from build123d import *

# Parameters (mm, degrees)
SKETCH1_W           = 820
SKETCH1_H           = 210
BOSS_EXTRUDE1_DEPTH = 210
CUT_EXTRUDE5_DEPTH  = 336
BOSS_EXTRUDE2_DEPTH = 210
BOSS_EXTRUDE3_DEPTH = 5
BOSS_EXTRUDE4_DEPTH = 5
SHELL2_START        = 5
SHELL2_DEPTH        = 200


# Read off the part's stored shape, not the designer's step: Shell2
with BuildPart() as part:
    # Sketch1 → Boss-Extrude1 (new body)
    with BuildSketch(Plane.XY):
        Rectangle(SKETCH1_W, SKETCH1_H)
    extrude(amount=BOSS_EXTRUDE1_DEPTH)

    # Sketch2 → Cut-Extrude5 (cut)
    with BuildSketch(Plane.XY.offset(210)):
        Polygon((-409.131759112, -82.443263164), (-310, -99.922866941), (-310, 99.822096903), (-310.868240888, 100.075961235), (-338.793852416, 105), (-410, 105), (-410, -82.367301929), align=None)
        Polygon((-410, -105), (-310, -105), (-410, -87.367301929), align=None)
    extrude(amount=-CUT_EXTRUDE5_DEPTH, mode=Mode.SUBTRACT)

    # Sketch6 → Boss-Extrude2 (add, through all)
    with BuildSketch(Plane.XY.offset(210)):
        Polygon((-338.793852416, 105), (-310.434120444, 105), (-410.434120444, 122.632698071), (-410.434120444, 117.555565011), (-311.302361333, 100.075961235), (-310.434120444, 99.437059413), (-310.434120444, 99.949029069), (-310.868240888, 100.075961235), align=None)
    extrude(amount=-BOSS_EXTRUDE2_DEPTH)

    # Sketch8 → Boss-Extrude3 (add)
    with BuildSketch(Plane.XY.offset(210)):
        Polygon((-410, -87.367301929), (-310, -105), (410, -105), (410, 105), (-310.434120444, 105), (-410.434120444, 122.632698071), align=None)
    extrude(amount=-BOSS_EXTRUDE3_DEPTH)

    # Sketch9 → Boss-Extrude4 (add)
    with BuildSketch(Plane(origin=(0, 0, 0), x_dir=(-1, 0, 0), z_dir=(0, 0, -1))):
        Polygon((310.434120444, 105), (310, -105), (410, -87.367301929), (410.434120444, 122.632698071), align=None)
    extrude(amount=-BOSS_EXTRUDE4_DEPTH)

    # Shell2 outline → Shell2 (cut)
    with BuildSketch(Plane.XY.offset(SHELL2_START)):
        Polygon((410, 100), (-310, 100), (-310, -99.922866941), (-309.562556682, -100), (410, -100), align=None)
    extrude(amount=SHELL2_DEPTH, mode=Mode.SUBTRACT)


solid = part.part
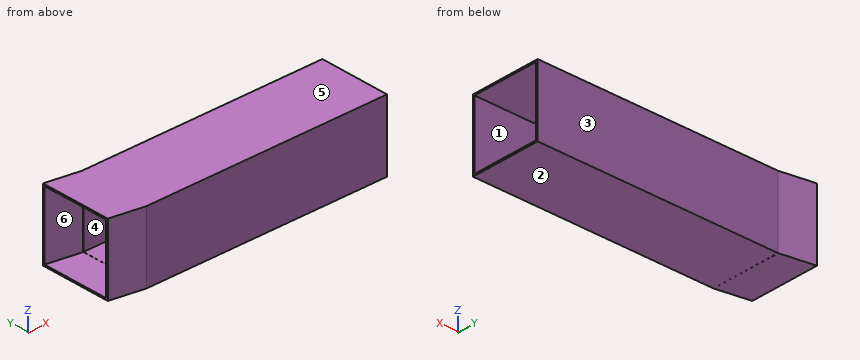
Model file for the job. Use its own axes, mm. Face numbers are marked on the shaded views. A direction names the side the tool comes from. Give positions to 0.01 mm unless a question says otherwise; leave off trailing zeros. Order: outer loops, then holes, each group sorted by start corner. A loop starts at its lowest first (then second) coordinate and runs counter-clockwise, first axis right, second up. Notation, with made-up numbers: M 25,9.5 L 31,9.5 A23 ccw 31,19.5 Z; hole C 18.25,-12 d11. An arc over 180 degrees is marked long. Write item = value, one per line.
Q1. Cut at A-A, the plane x = 134.5. List the corners of the cut face in (y, z), then the cut area to 3 significant figures.
Derived:
outline = M -105,0 L 105,0 L 105,210 L -105,210 Z; hole M -100,5 L 100,5 L 100,205 L -100,205 Z
area = 4,100 mm2
Q2. Two-plate mould, pull along Z, no slides. Class the marked faces 1, 2, 3 and 4: pulls with the +Z half, pulls with the -Z half, needs draft (parallel to the pull), parting line crosses it, or undercut.
Derived:
face_1 = undercut
face_2 = pulls with the -Z half
face_3 = needs draft
face_4 = undercut
Q3. Cut at D-D, the plane y = -58. List the corners of the cut face in (x, z).
Derived:
outline = M -410.06,0 L -310.1,0 L -310.1,5 L -410.06,5 Z; M -410.06,205 L 410,205 L 410,210 L -410.06,210 Z; M -310,0 L 410,0 L 410,5 L -310,5 Z
Q4. Cut at C-C, the plane z = 56. List the corners of the cut face in (x, y), then the cut area to 3 significant figures.
Derived:
outline = M -410.43,117.56 L -311.3,100.08 L -310.43,99.44 L -310.43,99.95 L -310,99.82 L -310,100 L 410,100 L 410,105 L -310.43,105 L -410.43,122.63 Z; M -410,-87.37 L -310,-105 L 410,-105 L 410,-100 L -309.56,-100 L -409.13,-82.44 L -410,-82.37 Z
area = 8,220 mm2
Q5. Drill centre lines: line 1 (Y direction, x = 78.5, z = 197); line 2 (Z direction, x = 220, y = -74). Where is each one in solid material? Low to high. Write a range as [from, to].
Derived:
line_1 = [-105, -100], [100, 105]
line_2 = [0, 5], [205, 210]
Q6. Cut at B-B, the plane y = 33. List the corners of the cut face in (x, z).
Derived:
outline = M -410.25,0 L -310.29,0 L -310.29,5 L -410.25,5 Z; M -410.25,205 L 410,205 L 410,210 L -410.25,210 Z; M -310,0 L 410,0 L 410,5 L -310,5 Z
Q7. Tool access for the marked faces 5 and 6: list every direction of +Z, -Z, +X, -X, +Y, -Y with a clear straight run to the whole face (end or side of a thin tool).
Derived:
face_5 = +Z, +X, -X, +Y, -Y
face_6 = -X
Q8. Flat gauge pins, fed straight in: pin 1 (5 mm diameter, centred on x = -278.5, z = 40, fed in from +Y); pin 2 (5.5 mm diameter, centred on y = -85, z = 147.5, fed in from -X); pin 3 (4 mm diameter, centred on y = -50, z = 2.5, fed in from -X). Where does each tip first touch, or does it go through?
Derived:
pin_1 = 105
pin_2 = -410
pin_3 = -410.08
